```python
from build123d import *

# Parameters (mm, degrees)
SKETCH_1_W                          = 43
SKETCH_1_H                          = 65
SM_BASE_FLANGE_1_DEPTH              = 0.8
SM_EDGE_FLANGE_1_STRIP_W            = 4.2
SM_EDGE_FLANGE_1_STRIP_H            = 0.8
SM_EDGE_FLANGE_1_STRIP_CUT_DEPTH    = 43
SM_EDGE_FLANGE_1_STRIP_2_W          = 4.2
SM_EDGE_FLANGE_1_STRIP_2_H          = 0.8
SM_EDGE_FLANGE_1_STRIP_CUT_2_DEPTH  = 43
SM_EDGE_FLANGE_1_DEPTH              = 43
SM_EDGE_FLANGE_1_BEND_DEPTH         = 43
SM_EDGE_FLANGE_2_STRIP_W            = 4.2
SM_EDGE_FLANGE_2_STRIP_H            = 0.8
SM_EDGE_FLANGE_2_STRIP_CUT_DEPTH    = 62.4
SM_EDGE_FLANGE_2_DEPTH              = 62.4
SM_EDGE_FLANGE_2_PROFILE_W          = 62.4
SM_EDGE_FLANGE_2_PROFILE_H          = 6.7
SM_EDGE_FLANGE_2_PROFILE_R          = 1.25
SM_EDGE_FLANGE_2_FLAT_DEPTH         = 0.8
SM_EDGE_FLANGE_3_STRIP_W            = 4.2
SM_EDGE_FLANGE_3_STRIP_H            = 0.8
SM_EDGE_FLANGE_3_STRIP_CUT_DEPTH    = 16
SM_EDGE_FLANGE_3_RELIEF_W           = 4.6
SM_EDGE_FLANGE_3_RELIEF_H           = 0.4
SM_EDGE_FLANGE_3_RELIEF_CUT_DEPTH   = 0.8
SM_EDGE_FLANGE_3_STRIP_2_W          = 4.2
SM_EDGE_FLANGE_3_STRIP_2_H          = 0.8
SM_EDGE_FLANGE_3_STRIP_CUT_2_DEPTH  = 16
SM_EDGE_FLANGE_3_RELIEF_2_W         = 4.6
SM_EDGE_FLANGE_3_RELIEF_2_H         = 0.4
SM_EDGE_FLANGE_3_RELIEF_CUT_2_DEPTH = 0.8
SM_EDGE_FLANGE_3_DEPTH              = 16
SM_EDGE_FLANGE_3_BEND_DEPTH         = 16
SKETCH_25_R                         = 3.25
EXTRUDE_1_DEPTH                     = 2
HOLE_WIZARD_M3_1_D                  = 2.5
HOLE_WIZARD_M3_1_DEPTH              = 2.8
FILLET_3_R                          = 5


# Sheet-metal steps are written as plain solids
with BuildPart() as part:
    # Sketch 1 → 基体-法兰1 (new body)
    with BuildSketch(Plane(origin=(0, 0, 0), x_dir=(1, 0, 0), z_dir=(0, 1, 0))):
        with Locations((21.5, 2.708940216)):
            Rectangle(SKETCH_1_W, SKETCH_1_H)
    extrude(amount=-SM_BASE_FLANGE_1_DEPTH)

    # 边线-法兰1 strip (across the edge) → 边线-法兰1 strip cut (cut)
    with BuildSketch(Plane(origin=(0, -0.8, -35.208940216), x_dir=(0, 0, 1), z_dir=(1, 0, 0))):
        with Locations((-0.8, -0.4)):
            Rectangle(SM_EDGE_FLANGE_1_STRIP_W, SM_EDGE_FLANGE_1_STRIP_H)
    extrude(amount=SM_EDGE_FLANGE_1_STRIP_CUT_DEPTH, mode=Mode.SUBTRACT)

    # 边线-法兰1 strip 2 (across the edge) → 边线-法兰1 strip cut 2 (cut)
    with BuildSketch(Plane(origin=(43, -0.8, 29.791059784), x_dir=(0, 0, -1), z_dir=(-1, 0, 0))):
        with Locations((-0.8, -0.4)):
            Rectangle(SM_EDGE_FLANGE_1_STRIP_2_W, SM_EDGE_FLANGE_1_STRIP_2_H)
    extrude(amount=SM_EDGE_FLANGE_1_STRIP_CUT_2_DEPTH, mode=Mode.SUBTRACT)

    # 边线-法兰1 section (across the edge) → 边线-法兰1 (add)
    with BuildSketch(Plane(origin=(0, -0.8, -35.208940216), x_dir=(0, 0, 1), z_dir=(1, 0, 0))):
        with BuildLine():
            Line((0, 0.5), (0, 22.2))
            Line((0, 22.2), (0.8, 22.2))
            Line((0.8, 22.2), (0.8, 0.5))
            ThreePointArc((0.8, 0.5), (0.946446609, 0.146446609), (1.3, 0))
            Line((1.3, 0), (1.3, -0.8))
            ThreePointArc((1.3, -0.8), (0.380761184, -0.419238816), (0, 0.5))
        make_face()
    extrude(amount=SM_EDGE_FLANGE_1_DEPTH)

    # 边线-法兰1 section 2 (across the edge) → 边线-法兰1 bend (add)
    with BuildSketch(Plane(origin=(43, -0.8, 29.791059784), x_dir=(0, 0, -1), z_dir=(-1, 0, 0))):
        with BuildLine():
            Line((0, 0.5), (0, 22.2))
            Line((0, 22.2), (0.8, 22.2))
            Line((0.8, 22.2), (0.8, 0.5))
            ThreePointArc((0.8, 0.5), (0.946446609, 0.146446609), (1.3, 0))
            Line((1.3, 0), (1.3, -0.8))
            ThreePointArc((1.3, -0.8), (0.380761184, -0.419238816), (0, 0.5))
        make_face()
    extrude(amount=SM_EDGE_FLANGE_1_BEND_DEPTH)

    # 边线-法兰2 strip (across the edge) → 边线-法兰2 strip cut (cut)
    with BuildSketch(Plane(origin=(0, -0.8, 28.491059784), x_dir=(1, 0, 0), z_dir=(0, 0, -1))):
        with Locations((-0.8, -0.4)):
            Rectangle(SM_EDGE_FLANGE_2_STRIP_W, SM_EDGE_FLANGE_2_STRIP_H)
    extrude(amount=SM_EDGE_FLANGE_2_STRIP_CUT_DEPTH, mode=Mode.SUBTRACT)

    # 边线-法兰2 bend section (across the edge) → 边线-法兰2 (add)
    with BuildSketch(Plane(origin=(0, -0.8, 28.491059784), x_dir=(1, 0, 0), z_dir=(0, 0, -1))):
        with BuildLine():
            Line((0, 0.5), (0.8, 0.5))
            ThreePointArc((0.8, 0.5), (0.946446609, 0.146446609), (1.3, 0))
            Line((1.3, 0), (1.3, -0.8))
            ThreePointArc((1.3, -0.8), (0.380761184, -0.419238816), (0, 0.5))
        make_face()
    extrude(amount=SM_EDGE_FLANGE_2_DEPTH)

    # 边线-法兰2 profile (on flange) → 边线-法兰2 flat (add)
    with BuildSketch(Plane(origin=(0, -0.8, 0), x_dir=(0, 0, -1), z_dir=(-1, 0, 0))):
        with Locations((2.708940216, 3.85)):
            Rectangle(SM_EDGE_FLANGE_2_PROFILE_W, SM_EDGE_FLANGE_2_PROFILE_H)
        with Locations((19.208940216, 4.2)):
            Circle(SM_EDGE_FLANGE_2_PROFILE_R, mode=Mode.SUBTRACT)
        with Locations((-13.791059784, 4.2)):
            Circle(SM_EDGE_FLANGE_2_PROFILE_R, mode=Mode.SUBTRACT)
    extrude(amount=-SM_EDGE_FLANGE_2_FLAT_DEPTH)

    # 边线-法兰3 strip (across the edge) → 边线-法兰3 strip cut (cut)
    with BuildSketch(Plane(origin=(0, -23, -34.408940216), x_dir=(0, 1, 0), z_dir=(1, 0, 0))):
        with Locations((-0.8, -0.4)):
            Rectangle(SM_EDGE_FLANGE_3_STRIP_W, SM_EDGE_FLANGE_3_STRIP_H)
    extrude(amount=SM_EDGE_FLANGE_3_STRIP_CUT_DEPTH, mode=Mode.SUBTRACT)

    # 边线-法兰3 relief (on the sheet) → 边线-法兰3 relief cut (cut)
    with BuildSketch(Plane(origin=(0, -21.7, -34.408940216), x_dir=(0, 1, 0), z_dir=(0, 0, 1))):
        with Locations((-1.9, -16.2)):
            Rectangle(SM_EDGE_FLANGE_3_RELIEF_W, SM_EDGE_FLANGE_3_RELIEF_H)
    extrude(amount=-SM_EDGE_FLANGE_3_RELIEF_CUT_DEPTH, mode=Mode.SUBTRACT)

    # 边线-法兰3 strip 2 (across the edge) → 边线-法兰3 strip cut 2 (cut)
    with BuildSketch(Plane(origin=(16, -23, 28.991059784), x_dir=(0, 1, 0), z_dir=(-1, 0, 0))):
        with Locations((-0.8, -0.4)):
            Rectangle(SM_EDGE_FLANGE_3_STRIP_2_W, SM_EDGE_FLANGE_3_STRIP_2_H)
    extrude(amount=SM_EDGE_FLANGE_3_STRIP_CUT_2_DEPTH, mode=Mode.SUBTRACT)

    # 边线-法兰3 relief 2 (on the sheet) → 边线-法兰3 relief cut 2 (cut)
    with BuildSketch(Plane(origin=(16, -21.7, 28.991059784), x_dir=(0, 1, 0), z_dir=(0, 0, -1))):
        with Locations((-1.9, 0.2)):
            Rectangle(SM_EDGE_FLANGE_3_RELIEF_2_W, SM_EDGE_FLANGE_3_RELIEF_2_H)
    extrude(amount=-SM_EDGE_FLANGE_3_RELIEF_CUT_2_DEPTH, mode=Mode.SUBTRACT)

    # 边线-法兰3 section (across the edge) → 边线-法兰3 (add)
    with BuildSketch(Plane(origin=(0, -23, -34.408940216), x_dir=(0, 1, 0), z_dir=(1, 0, 0))):
        with BuildLine():
            Line((0, 0.5), (0, 8))
            Line((0, 8), (0.8, 8))
            Line((0.8, 8), (0.8, 0.5))
            ThreePointArc((0.8, 0.5), (0.946446609, 0.146446609), (1.3, 0))
            Line((1.3, 0), (1.3, -0.8))
            ThreePointArc((1.3, -0.8), (0.380761184, -0.419238816), (0, 0.5))
        make_face()
    extrude(amount=SM_EDGE_FLANGE_3_DEPTH)

    # 边线-法兰3 section 2 (across the edge) → 边线-法兰3 bend (add)
    with BuildSketch(Plane(origin=(16, -23, 28.991059784), x_dir=(0, 1, 0), z_dir=(-1, 0, 0))):
        with BuildLine():
            Line((0, 0.5), (0, 8))
            Line((0, 8), (0.8, 8))
            Line((0.8, 8), (0.8, 0.5))
            ThreePointArc((0.8, 0.5), (0.946446609, 0.146446609), (1.3, 0))
            Line((1.3, 0), (1.3, -0.8))
            ThreePointArc((1.3, -0.8), (0.380761184, -0.419238816), (0, 0.5))
        make_face()
    extrude(amount=SM_EDGE_FLANGE_3_BEND_DEPTH)

    # 草图25 → 凸台-拉伸1 (add)
    with BuildSketch(Plane(origin=(0, -22.2, 0), x_dir=(1, 0, 0), z_dir=(0, 1, 0))):
        with Locations(Location((9, -24.791059784, 0), (0, 0, 270))):
            Circle(SKETCH_25_R)
        with Locations(Location((9, 30.208940216, 0), (0, 0, 270))):
            Circle(SKETCH_25_R)
    extrude(amount=EXTRUDE_1_DEPTH)

    # M3 螺纹孔1
    with Locations(Plane(origin=(0, -23, 0), x_dir=(-1, 0, 0), z_dir=(0, -1, 0))):
        with Locations((-9, -24.791059784), (-9, 30.208940216)):
            Hole(HOLE_WIZARD_M3_1_D / 2, depth=HOLE_WIZARD_M3_1_DEPTH)

    # 圆角3
    fillet_3_edges = [part.edges().sort_by_distance(p)[0] for p in [
        (0, -22.6, -26.408940216),
        (16, -22.6, -26.408940216),
        (16, -22.6, 20.991059784),
        (0, -22.6, 20.991059784),
    ]]
    fillet(fillet_3_edges, radius=FILLET_3_R)


solid = part.part
```
Design review of the part built by this model. Coordinates are the model's own, in mm. A direction names the side the tool comes from. Coordinates: 2 decimals unless noted, no trailing zeros. Order: outer loops, then holes, each group sorted by start corner. A loop starts at its lowest first (then second) coordinate and runs counter-clockwise, first axis right, second up.
1) Mouldability with a two-part tool opening along Y and no side actions: class faces 1 (the cylindrical face through (0.39, -3.78, 14.06)), 2 (the flat face through (22, 0, -3)), 3 (the flat face through (0, -5, -2)) as +Y half, -Y half, draft (parallel to the pull), parting line (faces both ways), or undercut.
2) Clearance check with flat-ended pins moving along their axes: pin 1 (2 mm diameter, centred on x = 13, z = 2.5, fed in from -Y); pin 2 (2 mm diameter, centred on y = -5, z = -19.21, fed in from -X); pin 3 (0.9 mm diameter, centred on x = 0.5, y = -0.5, fed in from +Z); pin 4 (6 mm diameter, centred on y = -8.5, z = -4, fed in from +X). State where each tip first meets the part, or that it passes through.
3) Take a section at A-A, the plane y = -3. Give the boundary of the cut face in (x, z).
4) Take a section at D-D, the plane z = -22. Give the boundary of the cut face in (x, y), and give its area (3 significant figures).
5) Wall thickness on line 1 along Z through (x, y) = (0.55, -5); line 2 along Z through (x, y) = (12, -20.5); line 3 along Y through (x, z) = (15, 26): over which ranges is each line inside the solid? List them lowest first.
6) For faces 4 (the cylindrical face through (7.75, -21.58, -30.26)), 5 (the flat face through (6, -22.2, -32)), 6 (the cylindrical face through (8.11, -22.61, 29.42)), 7 (the flat face through (9, -20.2, -28.8)), list the 3-axis set-ups (+Z, -Z, +X, -X, +Y, -Y) from which the entire face can be reached by the end or side of a thin tool; tool diameter is ignored.
7) Take a section at C-C, the plane x = 24. Give the boundary of the cut face in (y, z), and give its area (3 significant figures).
8) Take a section at B-B, the plane y = -12.5. Give the boundary of the cut face in (x, z).
Returned:
1. face 1: undercut
1. face 2: +Y half
1. face 3: draft
2. pin 1: stops at y = -0.8
2. pin 2: passes through
2. pin 3: stops at z = 29.74
2. pin 4: stops at x = 0.8
3. outline: (0, -35.21) - (43, -35.21) - (43, -34.41) - (0, -34.41) - close; (0, -33.91) - (0.8, -33.91) - (0.8, 28.49) - (0, 28.49) - close; (0, 28.99) - (43, 28.99) - (43, 29.79) - (0, 29.79) - close
4. outline: (0, -8) - (0.8, -8) - (0.8, -1.3) arc R0.5 cw to (1.3, -0.8) - (43, -0.8) - (43, 0) - (1.3, 0) arc R1.3 ccw to (0, -1.3) - close
4. area: 39.9 mm2
5. line 1: z = -35.21 to -34.41, -33.91 to -20.46, -17.96 to 12.54, 15.04 to 28.49, 28.99 to 29.79
5. line 2: z = -35.21 to -34.41, -31.46 to -28.96, 23.54 to 26.04, 28.99 to 29.79
5. line 3: y = -23 to -22.2, -0.8 to 0
6. face 4: -Y
6. face 5: none
6. face 6: +Z, -X, -Y
6. face 7: +X, -X
7. outline: (-23, -35.21) - (-1.3, -35.21) arc R1.3 ccw to (0, -33.91) - (0, 28.49) arc R1.3 ccw to (-1.3, 29.79) - (-23, 29.79) - (-23, 28.99) - (-1.3, 28.99) arc R0.5 cw to (-0.8, 28.49) - (-0.8, -33.91) arc R0.5 cw to (-1.3, -34.41) - (-23, -34.41) - close
7. area: 86.9 mm2
8. outline: (0, -35.21) - (43, -35.21) - (43, -34.41) - (0, -34.41) - close; (0, 28.99) - (43, 28.99) - (43, 29.79) - (0, 29.79) - close
